Can you work these out from the model? Positions are in its coordinate system, mm. Face numbers are marked on the shaded views. A direction names the side the tool comes from. Give positions to 0.01 mm unless a question says otherwise; leave off trailing zeros. Write each loop counter-clockwise with the first axis right and the second up, starting at its lowest first coordinate (ties: lowest second). Pieces come first, ordered by that corner, then holes. Notation, with made-up numbers: M 49,78 L 99,78 A15 ccw 99,101 Z; hole C 52,63.5 d10. An arc over 180 degrees is marked long. Write each question's results on one line, items separated by ' | '.
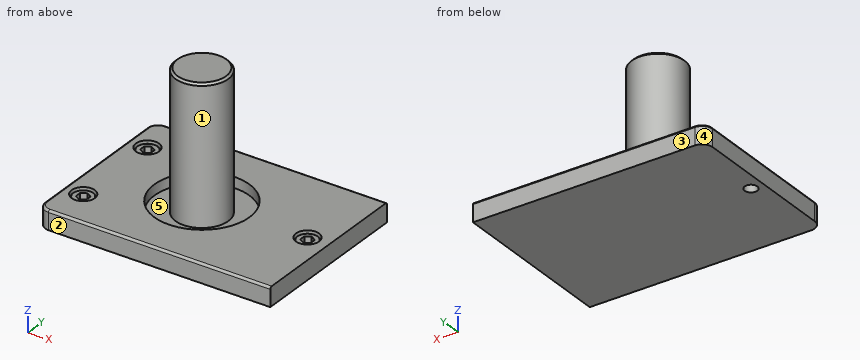
from build123d import *

# Parameters (mm, degrees)
BOSS_EXTRU_1_DEPTH               = 9
CONG_1_R                         = 1
ESQUISSE4_R                      = 5.5
ENL_V_MAT_EXTRU_1_DEPTH          = 7
ESQUISSE5_R                      = 5
BOSS_EXTRU_2_DEPTH               = 6
CONG_2_R                         = 0.5
ENL_V_MAT_EXTRU_2_DEPTH          = 4
R_P_TITION_LIN_AIRE1_COUNT       = 2
R_P_TITION_LIN_AIRE1_PITCH       = 44
CONG_2_OF_R_P_TITION_LIN_AIRE1_R = 0.5
ESQUISSE7_R                      = 5.5
ENL_V_MAT_EXTRU_3_DEPTH          = 7
ESQUISSE8_R                      = 5
BOSS_EXTRU_3_DEPTH               = 6
CONG_3_R                         = 0.5
ENL_V_MAT_EXTRU_4_DEPTH          = 5
ESQUISSE10_R                     = 3
ENL_V_MAT_EXTRU_5_DEPTH          = 5
ESQUISSE12_R                     = 22.5
ENL_V_MAT_EXTRU_7_DEPTH          = 5
ESQUISSE14_R                     = 12.5
BOSS_EXTRU_4_DEPTH               = 65
CHANFREIN1_SIZE                  = 1


with BuildPart() as part:
    # Esquisse1 → Boss.-Extru.1 (new body)
    with BuildSketch(Plane(origin=(0, 0, 0), x_dir=(-1, 0, 0), z_dir=(0, 0, 1))):
        with BuildLine():
            Line((0, 5), (0, 75))
            ThreePointArc((0, 75), (-1.464466094, 78.535533906), (-5, 80))
            Line((-5, 80), (-110, 80))
            Line((-110, 80), (-110, 0))
            Line((-110, 0), (-5, 0))
            ThreePointArc((-5, 0), (-1.464466094, 1.464466094), (0, 5))
        make_face()
    extrude(amount=BOSS_EXTRU_1_DEPTH)

    # Congé1
    cong_1_edges = [part.edges().sort_by_distance(p)[0] for p in [
        (1.464466094, -78.535533906, 9),
        (57.5, -80, 9),
        (57.5, 0, 9),
        (1.464466094, -1.464466094, 9),
        (0, -40, 9),
    ]]
    fillet(cong_1_edges, radius=CONG_1_R)

    # Esquisse4 → Enlèv. mat.-Extru.1 (cut)
    with BuildSketch(Plane.XY.offset(9)):
        with Locations((9, -18)):
            Circle(ESQUISSE4_R)
    enl_v_mat_extru_1 = extrude(amount=-ENL_V_MAT_EXTRU_1_DEPTH, mode=Mode.SUBTRACT)

    # Esquisse5 → Boss.-Extru.2 (add)
    with BuildSketch(Plane.XY.offset(2)):
        with Locations((9, -18)):
            Circle(ESQUISSE5_R)
    boss_extru_2 = extrude(amount=BOSS_EXTRU_2_DEPTH)

    # Congé2
    cong_2_edges = [part.edges().sort_by_distance(p)[0] for p in [
        (4, -18, 8),
    ]]
    fillet(cong_2_edges, radius=CONG_2_R)

    # Esquisse6 → Enlèv. mat.-Extru.2 (cut)
    with BuildSketch(Plane.XY.offset(8)):
        Polygon((9, -15.113248654), (6.5, -16.556624327), (6.5, -19.443375673), (9, -20.886751346), (11.5, -19.443375673), (11.5, -16.556624327), align=None)
    enl_v_mat_extru_2 = extrude(amount=-ENL_V_MAT_EXTRU_2_DEPTH, mode=Mode.SUBTRACT)

    # Répétition linéaire1: Enlèv. mat.-Extru.1, Boss.-Extru.2, Enlèv. mat.-Extru.2 ×2
    with Locations(*[(0, -i * R_P_TITION_LIN_AIRE1_PITCH, 0) for i in range(1, R_P_TITION_LIN_AIRE1_COUNT)]):
        add(enl_v_mat_extru_1, mode=Mode.SUBTRACT)
        add(boss_extru_2)
        add(enl_v_mat_extru_2, mode=Mode.SUBTRACT)

    # Congé2 of Répétition linéaire1
    cong_2_of_r_p_tition_lin_aire1_edges = [part.edges().sort_by_distance(p)[0] for p in [
        (4, -62, 8),
    ]]
    fillet(cong_2_of_r_p_tition_lin_aire1_edges, radius=CONG_2_OF_R_P_TITION_LIN_AIRE1_R)

    # Esquisse7 → Enlèv. mat.-Extru.3 (cut)
    with BuildSketch(Plane.XY.offset(9)):
        with Locations((100, -40)):
            Circle(ESQUISSE7_R)
    extrude(amount=-ENL_V_MAT_EXTRU_3_DEPTH, mode=Mode.SUBTRACT)

    # Esquisse8 → Boss.-Extru.3 (add)
    with BuildSketch(Plane.XY.offset(2)):
        with Locations((100, -40)):
            Circle(ESQUISSE8_R)
    extrude(amount=BOSS_EXTRU_3_DEPTH)

    # Congé3
    cong_3_edges = [part.edges().sort_by_distance(p)[0] for p in [
        (95, -40, 8),
    ]]
    fillet(cong_3_edges, radius=CONG_3_R)

    # Esquisse9 → Enlèv. mat.-Extru.4 (cut)
    with BuildSketch(Plane.XY.offset(8)):
        Polygon((100, -37.113248654), (97.5, -38.556624327), (97.5, -41.443375673), (100, -42.886751346), (102.5, -41.443375673), (102.5, -38.556624327), align=None)
    extrude(amount=-ENL_V_MAT_EXTRU_4_DEPTH, mode=Mode.SUBTRACT)

    # Esquisse10 → Enlèv. mat.-Extru.5 (cut)
    with BuildSketch(Plane(origin=(0, 0, 0), x_dir=(-1, 0, 0), z_dir=(0, 0, -1))):
        with Locations((-6, -40)):
            Circle(ESQUISSE10_R)
    extrude(amount=-ENL_V_MAT_EXTRU_5_DEPTH, mode=Mode.SUBTRACT)

    # Esquisse12 → Enlèv. mat.-Extru.7 (cut)
    with BuildSketch(Plane.XY.offset(9)):
        with Locations((50, -40)):
            Circle(ESQUISSE12_R)
    extrude(amount=-ENL_V_MAT_EXTRU_7_DEPTH, mode=Mode.SUBTRACT)

    # Esquisse14 → Boss.-Extru.4 (add)
    with BuildSketch(Plane.XY.offset(4)):
        with Locations((50, -40)):
            Circle(ESQUISSE14_R)
    extrude(amount=BOSS_EXTRU_4_DEPTH)

    # Chanfrein1
    chanfrein1_edges = [part.edges().sort_by_distance(p)[0] for p in [
        (37.5, -40, 69),
    ]]
    chamfer(chanfrein1_edges, length=CHANFREIN1_SIZE)


solid = part.part
Item 1: If I drill on line 1 (Y direction, x = 50, z = 5.1); line 2 (Y direction, x = 6, z = 4); line 3 (Y direction, x = 6, z = 1.25), over which ranges is the centre line in solid material (lowest first)? Write a range as from..to.
Geometry says:
line 1: y = -80..-62.5, -52.5..-27.5, -17.5..0 | line 2: y = -80..-66.61, -66..-58, -57.39..-43, -37..-22.61, -22..-14, -13.39..0 | line 3: y = -80..-43, -37..0
Item 2: I want a section at B-B, the plane y = -72. Please give me the cut outline in (x, z), and give its area (3 significant figures).
Geometry says:
outline: M 0,0 L 110,0 L 110,9 L 1,9 A1 ccw 0,8 Z | area: 990 mm2
Item 3: I want a section at D-D, the plane y = -26. Please give me the cut outline in (x, z), and give its area (3 significant figures).
Geometry says:
outline: M 0,0 L 110,0 L 110,9 L 67.61,9 L 67.61,4 L 32.39,4 L 32.39,9 L 1,9 A1 ccw 0,8 Z | area: 814 mm2
Item 4: I want a section at A-A, the plane x = 50. Please give me the cut outline in (y, z).
Geometry says:
outline: M -80,0 L 0,0 L 0,8 A1 ccw -1,9 L -17.5,9 L -17.5,4 L -27.5,4 L -27.5,68 L -28.5,69 L -51.5,69 L -52.5,68 L -52.5,4 L -62.5,4 L -62.5,9 L -79,9 A1 ccw -80,8 Z
Item 5: For the marked faces 1 and 2, which set-ups out of +Z, -Z, +X, -X, +Y, -Y let a thin tool reach every point of the face, with its end or its side?
Geometry says:
face 1: +Z | face 2: +Z, -Z, +X, -X, -Y
Item 6: I'm going to push flat-ended pins straight in: pin 1 (1.5 mm diameter, centred on x = 9.5, y = -18.5, fed in from +Z); pin 2 (1.8 mm diameter, centred on x = 5.5, y = -39, fed in from -Z); pin 3 (1.5 mm diameter, centred on x = 99, y = -41, fed in from +Z). Where does each tip first touch, or does it pass through?
Geometry says:
pin 1: stops at z = 4 | pin 2: stops at z = 5 | pin 3: stops at z = 3
Item 7: I want a section at C-C, the plane z = 12.5. Please give me the cut outline in (x, y).
Geometry says:
outline: C 50,-40 d25
Item 8: Thinking about a two-plate mould opening in X: for the marked faces 3, 4 and 5, which applies, +X half, -X half, draft (parallel to the pull), parting line (faces both ways), or undercut?
Geometry says:
face 3: draft | face 4: -X half | face 5: undercut
